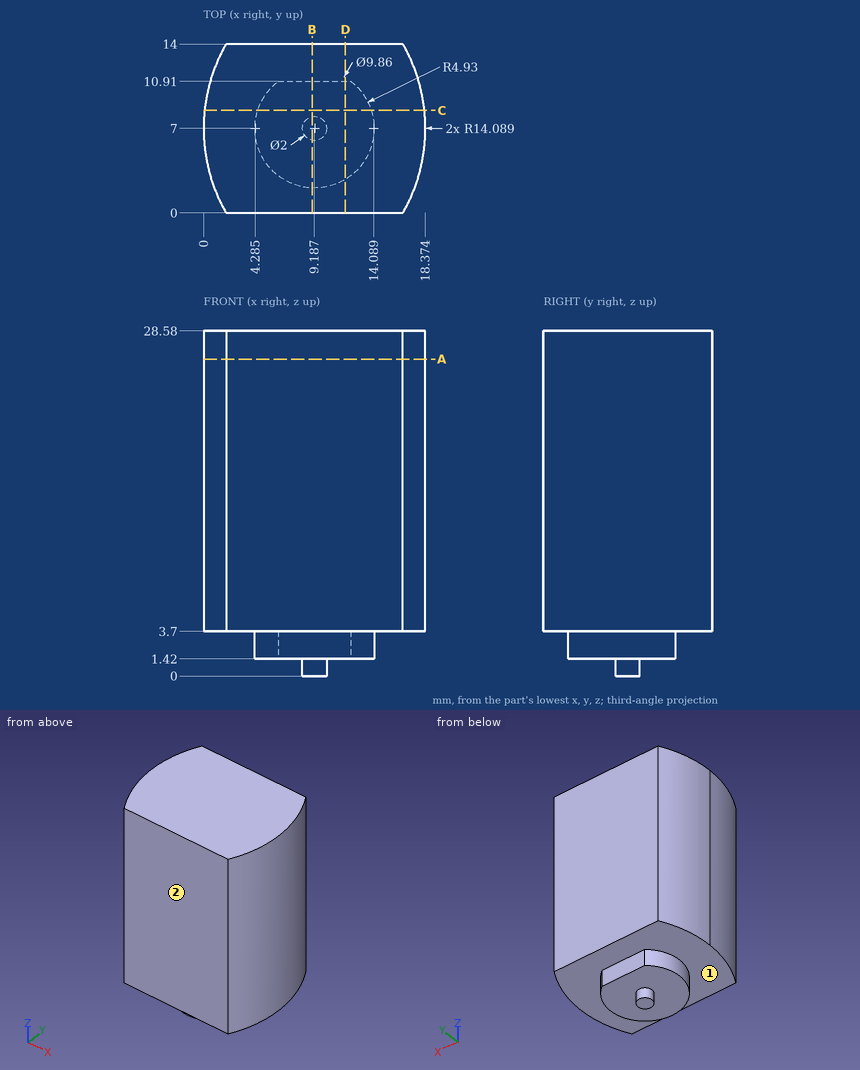
Check sheet for the drawn part. Datum: minimum x, y, z corner. Units: mm. A direction names the side the tool comes from. Round coordinates to 2 decimals unless told otherwise and drop trailing zeros. Order: outer loops, then holes, each group sorted by start corner. A loop starts at its lowest first (then second) coordinate and runs counter-clockwise, first axis right, second up. Notation, with made-up numbers: (-34, 39) -> (15, 39) arc R13 ccw to (15, 44) -> close; hole circle Ø6 at (0.25, 25). An arc over 180 degrees is marked (long way). Put each result on its own line as item: value. Start each with the question number.
(1) Material ranges on line 1 along Z through (x, y) = (5.5, 4.75); line 2 along Z through (x, y) = (14.5, 6.25); line 3 along X through (y, z) = (8.5, 22.5) (1 decimal), recorded low to high.
(2) Depth check by flat-ended pin: pin 1 Ø1 at (x, y) = (16.5, 7) entering from -Z; pin 2 Ø4 at (x, y) = (11, 9) entering from -Z; pin 3 Ø4 at (y, z) = (3.5, 12) entering from +X (1 decimal); pin 4 Ø0.7 at (x, z) = (9.5, 2.5) entering from +Y. Enter the tip coordinate at first touch or a pass-through.
(3) Tool access check on the marked faces 1 and 2. Record the directions out of +Z, -Z, +X, -X, +Y, -Y that give a thin tool (end or side, any length) a straight path to the whole face; none if there is none.
(4) Section check C-C (y = 8.5). Enter the section's corners in (x, z) (1 decimal).
(5) Section check A-A (z = 26.25). Enter the section's corners in (x, y) (1 decimal).
(6) Section check D-D (x = 11.75). Enter the section's corners in (y, z), then the cut area to 3 significant figures.
(7) Section check B-B (x = 9). Enter the section's corners in (y, z).
Completed:
1. line 1: z = 1.42 to 28.58
1. line 2: z = 3.7 to 28.58
1. line 3: x = 0.1 to 18.3
2. pin 1: stops at z = 3.7
2. pin 2: stops at z = 0
2. pin 3: stops at x = 18.3
2. pin 4: stops at y = 10.91
3. face 1: -Z
3. face 2: +Z, -Z, +X, -X, -Y
4. outline: (0.1, 3.7) -> (4.5, 3.7) -> (4.5, 1.4) -> (13.9, 1.4) -> (13.9, 3.7) -> (18.3, 3.7) -> (18.3, 28.6) -> (0.1, 28.6) -> close
5. outline: (1.9, 0) -> (16.5, 0) arc R14.1 ccw to (16.5, 14) -> (1.9, 14) arc R14.1 ccw to start
6. outline: (0, 3.7) -> (2.79, 3.7) -> (2.79, 1.42) -> (10.91, 1.42) -> (10.91, 3.7) -> (14, 3.7) -> (14, 28.58) -> (0, 28.58) -> close
6. area: 367 mm2
7. outline: (0, 3.7) -> (2.07, 3.7) -> (2.07, 1.42) -> (6.02, 1.42) -> (6.02, 0) -> (7.98, 0) -> (7.98, 1.42) -> (10.91, 1.42) -> (10.91, 3.7) -> (14, 3.7) -> (14, 28.58) -> (0, 28.58) -> close
